The model under review builds one solid part; all positions refer to its coordinate system, in mm. Face numbers are marked on the shaded views. Coordinates: 2 decimals unless noted, no trailing zeros. Write each loop counter-clockwise with the first axis right and the second up, starting at its lowest first coordinate (ties: lowest second). Pieces come first, ordered by that corner, then holes.
1) Add section C-C, the plane x = 35. State the section outline as (y, z) points, then the cut area to 3 significant figures.
2) Add section D-D, the plane y = -4.5. State the section outline as (x, z) points, then the cut area to 3 significant figures.
3) Add section B-B, the plane z = 64. State the section outline as (x, y) points, then the cut area to 3 significant figures.
4) Mouldability with a two-part tool opening along Z and no side actions: class the marked faces 1, 2 and 3 as released by +Z, released by -Z, zero draft, split by the parting line, or undercut.
5) Add section A-A, the plane y = -23. State the section outline as (x, z) points.
6) For line 1 (X direction, y = -18, z = 57); line 2 (X direction, y = -17, z = 63.5); line 3 (X direction, y = -9, z = 22), list the stretches that pass through material, from the lowest coordinate up.
7) For P1, Ø12, axis at x = -24.5, y = -17.5, coming from the -Z side; P2, Ø1.6, axis at x = -23, y = -20.5, coming from the -Z side; P3, Ø2, axis at x = 1, z = -14.5, coming from the +Y side; P4, Ø12, axis at x = 25.5, y = -8, coming from the +Z side, all flat-tipped, find the tip position at first contact; note any pin that passes through.
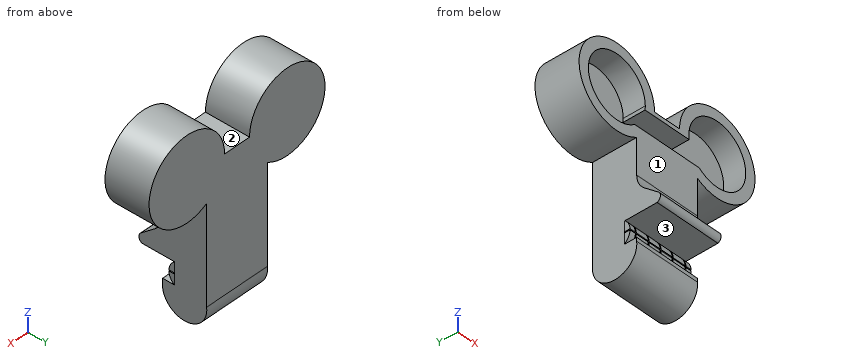
from build123d import *

# Parameters (mm, degrees)
F1_DEPTH  = 25.4
F3_DEPTH  = 38.1
F5_DEPTH  = 38.1
F4_W      = 6.9873932093
F4_H      = 12.5755788758
F6_DEPTH  = 74.2380387742
F10_DEPTH = 19.1516
F12_DEPTH = 12.7
F14_W     = 3.3459962718
F14_H     = 0.297806253
F14_W_2   = 0.595612506
F14_W_3   = 7.4709270083
F14_H_2   = 5.9899831849
F14_W_4   = 6.8456454549
F14_W_5   = 6.9815108719
F14_W_6   = 7.4240169587
F14_W_7   = 3.2570409043
F15_DEPTH = 3.2512
F16_R     = 11.8404858978


with BuildPart() as f1:
    # F0 (on Front) → F1 (new body)
    with BuildSketch(Plane.XZ):
        with BuildLine():
            Line((1.8669807536, 56.3211729646), (-13.7737724727, 56.3211729646))
            ThreePointArc((-13.7737724727, 56.3211729646), (-58.1397054496, 67.8494936223), (-24.9982573971, 36.1811717994))
            Line((-24.9982573971, 36.1811717994), (-24.9982573971, -19.8788270354))
            Line((-24.9982573971, -19.8788270354), (13.1017426029, -19.8788270354))
            Line((13.1017426029, -19.8788270354), (13.1017426029, 36.1748193053))
            ThreePointArc((13.1017426029, 36.1748193053), (46.2299722184, 67.8547699704), (1.8669807536, 56.3211729646))
        make_face()
        with BuildLine():
            ThreePointArc((-26.1908572696, 42.4751723279), (-53.0432504616, 65.0145085437), (-19.7552210705, 54.0154269254))
            Line((-19.7552210705, 54.0154269254), (7.8484293514, 54.0154269254))
            ThreePointArc((7.8484293514, 54.0154269254), (41.1364587425, 65.0145085437), (14.2840655504, 42.4751723279))
            Line((14.2840655504, 42.4751723279), (-26.1908572696, 42.4751723279))
        make_face(mode=Mode.SUBTRACT)
        with BuildLine():
            Line((7.8484293514, 54.0154269254), (-19.7552210705, 54.0154269254))
            ThreePointArc((-19.7552210705, 54.0154269254), (-53.0432504616, 65.0145085437), (-26.1908572696, 42.4751723279))
            Line((-26.1908572696, 42.4751723279), (14.2840655504, 42.4751723279))
            ThreePointArc((14.2840655504, 42.4751723279), (41.1364587425, 65.0145085437), (7.8484293514, 54.0154269254))
        make_face()
    extrude(amount=F1_DEPTH)

    # F2 (on face) → F3 (join, through all)
    with BuildSketch(Plane.YZ.offset(13.1017426029)):
        with BuildLine():
            Line((0, -19.8788270354), (-25.4, -19.8788270354))
            ThreePointArc((-25.4, -19.8788270354), (-12.7, -34.0406843529), (0, -19.8788270354))
        make_face()
    extrude(amount=-F3_DEPTH)

    # F4 (on face) → F5 (join, through all)
    with BuildSketch(Plane.YZ.offset(13.1017426029)):
        with BuildLine():
            Line((-25.4, -5.1776664332), (-25.4, 10.2089252323))
            Line((-25.4, 10.2089252323), (-37.9417426884, 0))
            ThreePointArc((-37.9417426884, 0), (-39.036129938, -2.7980343054), (-37.202000618, -5.1776664332))
            Line((-37.202000618, -5.1776664332), (-25.4, -5.1776664332))
        make_face()
    extrude(amount=-F5_DEPTH)

    # F4 (on face) → F6 (cut, through all)
    with BuildSketch(Plane.YZ.offset(13.1017426029)):
        with Locations((-21.9063033953, -11.4654558711)):
            Rectangle(F4_W, F4_H)
    extrude(amount=-F6_DEPTH, mode=Mode.SUBTRACT)

    # F9 (on line) → F10 (join, symmetric)
    with BuildSketch(Plane(origin=(-5.9482573971, 0, 0), x_dir=(0, -1, 0), z_dir=(-1, 0, 0))):
        with BuildLine():
            ThreePointArc((18.4126067907, -17.753245309), (21.6845212051, -11.4654558711), (18.4126067907, -5.1776664332))
            Line((18.4126067907, -5.1776664332), (18.4126067907, -17.753245309))
        make_face()
    extrude(amount=F10_DEPTH, both=True)

    # F11 (on face) → F12 (cut)
    with BuildSketch(Plane.XZ.offset(25.4)):
        with BuildLine():
            Line((-26.1908572696, 42.4751723279), (-24.9982573971, 42.4751723279))
            Line((-24.9982573971, 42.4751723279), (13.1017426029, 42.4751723279))
            Line((13.1017426029, 42.4751723279), (14.2840655504, 42.4751723279))
            ThreePointArc((14.2840655504, 42.4751723279), (41.6664593623, 63.9872752599), (7.6988727683, 56.3211729646))
            ThreePointArc((7.6988727683, 56.3211729646), (7.736301157, 55.1658773348), (7.8484293514, 54.0154269254))
            Line((7.8484293514, 54.0154269254), (-19.7552210705, 54.0154269254))
            ThreePointArc((-19.7552210705, 54.0154269254), (-19.6430928761, 55.1658773348), (-19.6056644874, 56.3211729646))
            ThreePointArc((-19.6056644874, 56.3211729646), (-53.5732510815, 63.9872752599), (-26.1908572696, 42.4751723279))
        make_face()
    extrude(amount=-F12_DEPTH, mode=Mode.SUBTRACT)

    # F14 (on line) → F15 (cut)
    with BuildSketch(Plane.XZ.offset(21.6845212051)):
        with Locations((-23.4268592612, -11.3165527446)):
            Rectangle(F14_W, F14_H)
        with Locations((-23.4268592612, -11.6143589976)):
            Rectangle(F14_W, F14_H)
        with Locations((-21.4560548723, -11.3165527446)):
            Rectangle(F14_W_2, F14_H)
        with Locations((-21.4560548723, -11.6143589976)):
            Rectangle(F14_W_2, F14_H)
        with Locations((-17.4227851151, -11.3165527446)):
            Rectangle(F14_W_3, F14_H)
        with Locations((-17.4227851151, -11.6143589976)):
            Rectangle(F14_W_3, F14_H)
        with Locations((-21.4560548723, -8.1726580256)):
            Rectangle(F14_W_2, F14_H_2)
        with Locations((-21.4560548723, -14.7582537165)):
            Rectangle(F14_W_2, F14_H_2)
        with Locations((-13.389515358, -11.3165527446)):
            Rectangle(F14_W_2, F14_H)
        with Locations((-13.389515358, -11.6143589976)):
            Rectangle(F14_W_2, F14_H)
        with Locations((-9.6688863776, -11.3165527446)):
            Rectangle(F14_W_4, F14_H)
        with Locations((-9.6688863776, -11.6143589976)):
            Rectangle(F14_W_4, F14_H)
        with Locations((-13.389515358, -8.1726580256)):
            Rectangle(F14_W_2, F14_H_2)
        with Locations((-13.389515358, -14.7582537165)):
            Rectangle(F14_W_2, F14_H_2)
        with Locations((-5.9482573971, -11.3165527446)):
            Rectangle(F14_W_2, F14_H)
        with Locations((-5.9482573971, -11.6143589976)):
            Rectangle(F14_W_2, F14_H)
        with Locations((-2.1596957082, -11.3165527446)):
            Rectangle(F14_W_5, F14_H)
        with Locations((-2.1596957082, -11.6143589976)):
            Rectangle(F14_W_5, F14_H)
        with Locations((-5.9482573971, -8.1726580256)):
            Rectangle(F14_W_2, F14_H_2)
        with Locations((-5.9482573971, -14.7582537165)):
            Rectangle(F14_W_2, F14_H_2)
        with Locations((1.6288659808, -11.3165527446)):
            Rectangle(F14_W_2, F14_H)
        with Locations((1.6288659808, -11.6143589976)):
            Rectangle(F14_W_2, F14_H)
        with Locations((5.6386807132, -11.3165527446)):
            Rectangle(F14_W_6, F14_H)
        with Locations((5.6386807132, -11.6143589976)):
            Rectangle(F14_W_6, F14_H)
        with Locations((1.6288659808, -8.1726580256)):
            Rectangle(F14_W_2, F14_H_2)
        with Locations((1.6288659808, -14.7582537165)):
            Rectangle(F14_W_2, F14_H_2)
        with Locations((9.6484954455, -11.3165527446)):
            Rectangle(F14_W_2, F14_H)
        with Locations((9.6484954455, -11.6143589976)):
            Rectangle(F14_W_2, F14_H)
        with Locations((11.5748221507, -11.3165527446)):
            Rectangle(F14_W_7, F14_H)
        with Locations((11.5748221507, -11.6143589976)):
            Rectangle(F14_W_7, F14_H)
        with Locations((9.6484954455, -8.1726580256)):
            Rectangle(F14_W_2, F14_H_2)
        with Locations((9.6484954455, -14.7582537165)):
            Rectangle(F14_W_2, F14_H_2)
    extrude(amount=-F15_DEPTH, mode=Mode.SUBTRACT)

    # F16
    f16_edges = [f1.edges().sort_by_distance(p)[0] for p in [
        (-5.948257, -25.4, 10.208925),
    ]]
    fillet(f16_edges, radius=F16_R)


solid = f1.part
Geometry results:
1. outline: (-25.4, 34.61) - (0, 34.61) - (0, 78.03) - (-25.4, 78.03) - (-25.4, 71.46) - (-12.7, 71.46) - (-12.7, 41.18) - (-25.4, 41.18) - close
1. area: 718 mm2
2. outline: (-25, -31.06) - (13.1, -31.06) - (13.1, 36.17) arc R23.68 ccw (long way) to (1.87, 56.32) - (-13.77, 56.32) arc R23.68 ccw (long way) to (-25, 36.18) - close
2. area: 6,530 mm2
3. outline: (-59.86, -25.4) - (-53.57, -25.4) - (-53.57, -12.7) - (-21.34, -12.7) - (-21.34, -25.4) - (-15.05, -25.4) - (-15.05, 0) - (-59.86, 0) - close; (3.15, -25.4) - (9.44, -25.4) - (9.44, -12.7) - (41.66, -12.7) - (41.66, -25.4) - (47.95, -25.4) - (47.95, 0) - (3.15, 0) - close
3. area: 1,460 mm2
4. face 1: zero draft
4. face 2: released by +Z
4. face 3: undercut
5. outline: (-25, -28.82) - (13.1, -28.82) - (13.1, -17.75) - (-25, -17.75) - close; (-25, -5.18) - (13.1, -5.18) - (13.1, 36.17) arc R23.68 ccw (long way) to (1.87, 56.32) - (-13.77, 56.32) arc R23.68 ccw (long way) to (-25, 36.18) - close; hole (-26.19, 42.48) - (14.28, 42.48) arc R17.85 ccw (long way) to (7.85, 54.02) - (-19.76, 54.02) arc R17.85 ccw (long way) to start
6. line 1: x = -61.13 to -55.29, -19.62 to -13.78, 1.88 to 7.71, 43.38 to 49.22
6. line 2: x = -60.02 to -53.8, -21.11 to -14.89, 2.98 to 9.21, 41.89 to 48.11
6. line 3: x = -25 to 13.1
7. P1: stops at z = -34.04
7. P2: stops at z = -31.95
7. P3: stops at y = 0
7. P4: stops at z = 80
